For this review, take the finished solid that the model builds, in its own axes (mm). Coordinates: 2 decimals unless noted, no trailing zeros. Order: outer loops, then holes, each group sorted by start corner. A loop starts at its lowest first (then second) coordinate and runs counter-clockwise, first axis right, second up. Notation, with made-up numbers: (-9, 3) -> (8, 3) arc R18 ccw to (8, 20) -> close; hole circle Ø1 at (-30.75, -11). An arc over 180 degrees is marked (long way). Write item = value, one per line. Start each with the question number.
1) Wall thickness on probe 1 along Y at (x, z) = (30, 1.15); probe 2 along X at (y, z) = (-56.5, 0.1); probe 3 along Y at (x, z) = (13.5, 1): over which ranges is each line inside the solid? List them lowest first. Write a range as [from, to].
2) Insertion check: pin 1 Ø0.9 at (y, z) = (-62.5, 1) entering from -X; pin 2 Ø0.9 at (y, z) = (-21, 1.5) entering from +X; pin 3 Ø3 at (x, y) = (17.5, -11.5) entering from -Z; pin 4 Ø1.5 at (x, z) = (39, 1) entering from +Y. Each pin has a flat end and moves straight along its axis. Give the tip position at first contact, or say it passes through.
3) Consider section C-C on y = 0. Give the boundary of the cut face in (x, z), and give its area (3 significant figures).
4) Consider section A-A on x = -30. Give the boundary of the cut face in (y, z).
5) Consider section B-B on z = 1.95. Give the boundary of the cut face in (x, y), and give its area (3 significant figures).
6) Consider section D-D on y = -68.5. Give the boundary of the cut face in (x, z).
from build123d import *

# Parameters (mm, degrees)
SKETCH1_R           = 2
BOSS_EXTRUDE1_DEPTH = 3
SKETCH2_W           = 3
SKETCH2_H           = 96
CUT_EXTRUDE1_DEPTH  = 10
SKETCH3_W           = 3
SKETCH3_H           = 10
BOSS_EXTRUDE2_DEPTH = 3


with BuildPart() as part:
    # Sketch1 → Boss-Extrude1 (new body)
    with BuildSketch(Plane.XY):
        Polygon((5, 8.25), (40, 8.25), (40, -31.75), (37, -31.75), (37, -41.75), (40, -41.75), (40, -81.75), (5, -81.75), (5, -84.75), (-5, -84.75), (-5, -81.75), (-40, -81.75), (-40, -41.75), (-37, -41.75), (-37, -31.75), (-40, -31.75), (-40, 8.25), (-5, 8.25), (-5, 11.25), (5, 11.25), align=None)
        with Locations((30, 0)):
            Circle(SKETCH1_R, mode=Mode.SUBTRACT)
        with Locations(Location((30, -73.5, 0), (0, 0, 180))):
            Circle(SKETCH1_R, mode=Mode.SUBTRACT)
        with Locations((-30, -73.5)):
            Circle(SKETCH1_R, mode=Mode.SUBTRACT)
        with Locations(Location((-30, 0, 0), (0, 0, 180))):
            Circle(SKETCH1_R, mode=Mode.SUBTRACT)
    extrude(amount=BOSS_EXTRUDE1_DEPTH)

    # Sketch2 → Cut-Extrude1 (cut)
    with BuildSketch(Plane.XY.offset(3)):
        with Locations((38.5, -36.75)):
            Rectangle(SKETCH2_W, SKETCH2_H)
        with Locations((-38.5, -36.75)):
            Rectangle(SKETCH2_W, SKETCH2_H)
    extrude(amount=-CUT_EXTRUDE1_DEPTH, mode=Mode.SUBTRACT)

    # Sketch3 → Boss-Extrude2 (add)
    with BuildSketch(Plane.XY.offset(3)):
        with Locations((38.5, -36.75)):
            Rectangle(SKETCH3_W, SKETCH3_H)
        with Locations((-38.5, -36.75)):
            Rectangle(SKETCH3_W, SKETCH3_H)
    extrude(amount=-BOSS_EXTRUDE2_DEPTH)


solid = part.part
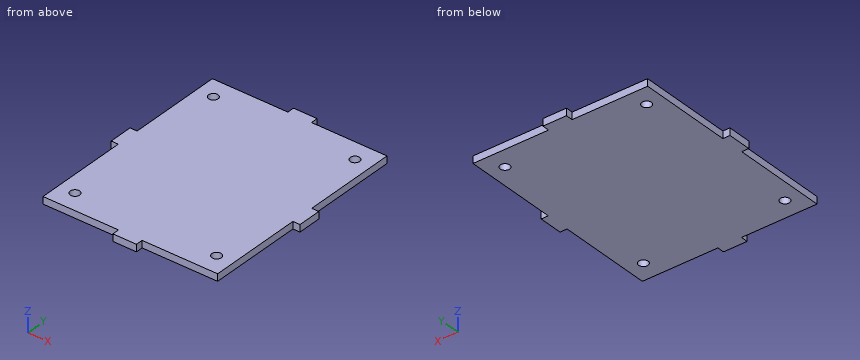
Answer sheet:
q1.probe_1 = [-81.75, -75.5], [-71.5, -2], [2, 8.25]
q1.probe_2 = [-37, 37]
q1.probe_3 = [-81.75, 8.25]
q2.pin_1 = -37
q2.pin_2 = 37
q2.pin_3 = 0
q2.pin_4 = -31.75
q3.outline = (-37, 0) -> (-32, 0) -> (-32, 3) -> (-37, 3) -> close; (-28, 0) -> (28, 0) -> (28, 3) -> (-28, 3) -> close; (32, 0) -> (37, 0) -> (37, 3) -> (32, 3) -> close
q3.area = 198 mm2
q4.outline = (-81.75, 0) -> (-75.5, 0) -> (-75.5, 3) -> (-81.75, 3) -> close; (-71.5, 0) -> (-2, 0) -> (-2, 3) -> (-71.5, 3) -> close; (2, 0) -> (8.25, 0) -> (8.25, 3) -> (2, 3) -> close
q5.outline = (-40, -41.75) -> (-37, -41.75) -> (-37, -81.75) -> (-5, -81.75) -> (-5, -84.75) -> (5, -84.75) -> (5, -81.75) -> (37, -81.75) -> (37, -41.75) -> (40, -41.75) -> (40, -31.75) -> (37, -31.75) -> (37, 8.25) -> (5, 8.25) -> (5, 11.25) -> (-5, 11.25) -> (-5, 8.25) -> (-37, 8.25) -> (-37, -31.75) -> (-40, -31.75) -> close; hole circle Ø4 at (-30, -73.5); hole circle Ø4 at (-30, 0); hole circle Ø4 at (30, -73.5); hole circle Ø4 at (30, 0)
q5.area = 6,730 mm2
q6.outline = (-37, 0) -> (37, 0) -> (37, 3) -> (-37, 3) -> close
